Can you work these out from the drawing? Everything is in mm from the part's minimum corner. A direction names the side the tool comes from. Round coordinates to 2 decimals unless told otherwise and drop trailing zeros. Loops run counter-clockwise (first coordinate to the right, second up) from the corner with the lowest first, then second, coordinate; pieces in that order, holes last. Notation, with made-up numbers: M 54.25,64 L 112.25,64 A26 cw 112.25,97 Z; hole C -30.5,3.5 d7. An arc over 180 degrees is marked long. Use a Markdown table: item, result.
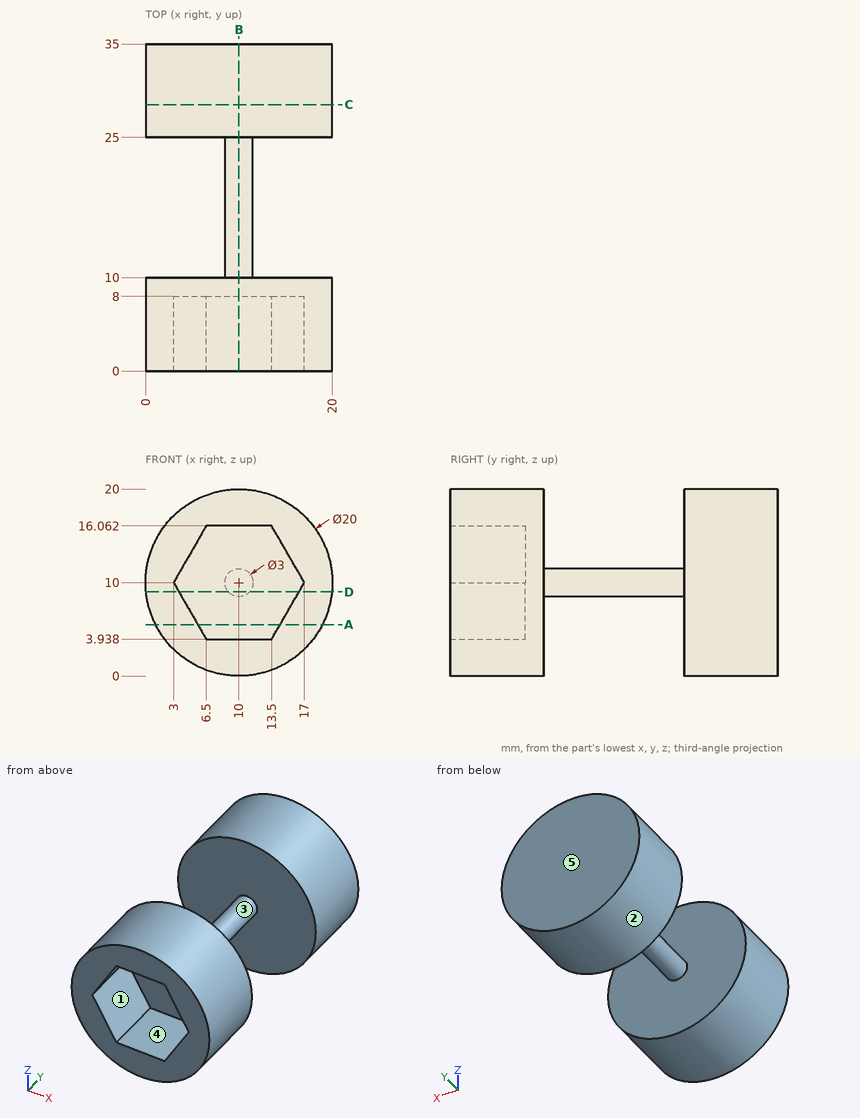
1. I need wall thicknesses on probe 1 along Y at (x, z) = (18, 13); probe 2 along Y at (x, z) = (9, 15.75); probe 3 along Z at (x, y) = (15.75, 3.5) (1 decimal). Which ranges of each line are inside material? Lowest first, please. Write a range as from..to.
Answer sheet:
| item | result |
|---|---|
| probe 1 | 0..10, 25..35 |
| probe 2 | 8..10, 25..35 |
| probe 3 | 1.8..7.8, 12.2..18.2 |
2. Imagine slicing it at A-A, the plane z = 5.5. Write out the boundary of the cut face in (x, y).
Answer sheet:
| item | result |
|---|---|
| outline | M 1.07,0 L 5.6,0 L 5.6,8 L 14.4,8 L 14.4,0 L 18.93,0 L 18.93,10 L 1.07,10 Z; M 1.07,25 L 18.93,25 L 18.93,35 L 1.07,35 Z |
3. Imagine slicing it at B-B, the plane x = 10. Write out the boundary of the cut face in (y, z).
Answer sheet:
| item | result |
|---|---|
| outline | M 0,0 L 10,0 L 10,8.5 L 25,8.5 L 25,0 L 35,0 L 35,20 L 25,20 L 25,11.5 L 10,11.5 L 10,20 L 0,20 L 0,16.06 L 8,16.06 L 8,3.94 L 0,3.94 Z |
4. Imagine slicing it at C-C, the plane y = 28.5. Write out the boundary of the cut face in (x, z), then the cut area to 3 significant figures.
Answer sheet:
| item | result |
|---|---|
| outline | C 10,10 d20 |
| area | 314 mm2 |
5. For pin 1 Ø3.5 at (x, z) = (9, 12.5) entering from -Y; pin 2 Ø2 at (x, y) = (17.5, 23) entering from +Z; pin 3 Ø5 at (x, y) = (16.5, 28) entering from +Z (1 decimal); pin 4 Ø10 at (x, y) = (6.5, 16) entering from +Z, each with a flat end and sliding along its axis, tell me the tip position at first contact or that it passes through.
Answer sheet:
| item | result |
|---|---|
| pin 1 | y = 8 |
| pin 2 | through |
| pin 3 | z = 19.2 |
| pin 4 | z = 11.5 |
6. Which directions (+Z, -Z, +X, -X, +Y, -Y) give clear straight access to the entire face, cutting with the end or side of a thin tool? Please do the marked faces 1 and 2.
Answer sheet:
| item | result |
|---|---|
| face 1 | -Y |
| face 2 | +Y, -Y |
7. Imagine slicing it at D-D, the plane z = 9. Write out the boundary of the cut face in (x, y).
Answer sheet:
| item | result |
|---|---|
| outline | M 0.05,0 L 3.58,0 L 3.58,8 L 16.42,8 L 16.42,0 L 19.95,0 L 19.95,10 L 11.12,10 L 11.12,25 L 19.95,25 L 19.95,35 L 0.05,35 L 0.05,25 L 8.88,25 L 8.88,10 L 0.05,10 Z |
8. We'd pull the mould along Y, two halves only. Please class the marked faces 3, 4 and 5: +Y half, -Y half, draft (parallel to the pull), parting line (faces both ways), or undercut.
Answer sheet:
| item | result |
|---|---|
| face 3 | undercut |
| face 4 | draft |
| face 5 | +Y half |
